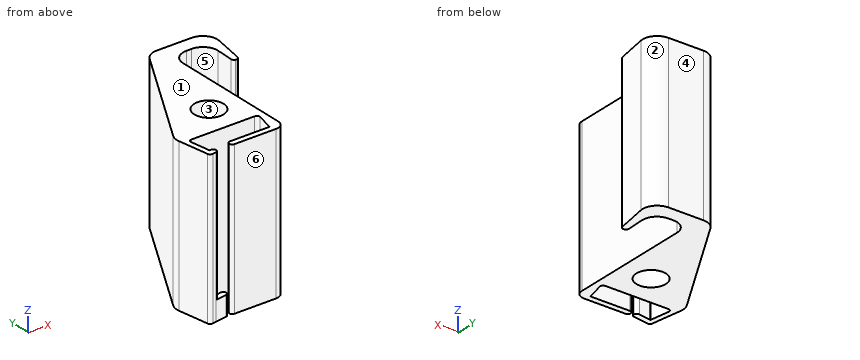
from build123d import *

# Parameters (mm, degrees)
F0_R     = 6.35
F1_DEPTH = 66.04
F3_DEPTH = 8.509


with BuildPart() as f1:
    # F0 (on Top) → F1 (new body)
    with BuildSketch(Plane.XY):
        with BuildLine():
            ThreePointArc((-22.546312, -25.022118), (-22.038436, -25.850898), (-21.093276, -26.077811))
            Line((-21.093276, -26.077811), (-19.546685, -25.832855))
            ThreePointArc((-19.546685, -25.832855), (-18.717905, -25.324978), (-18.490992, -24.379819))
            ThreePointArc((-18.490992, -24.379819), (-18.998869, -23.551039), (-19.944028, -23.324126))
            Line((-19.944028, -23.324126), (-20.432482, -23.40149))
            Line((-20.432482, -23.40149), (-21.789241, -14.835248))
            ThreePointArc((-21.789241, -14.835248), (-21.500592, -13.811777), (-20.534877, -13.366576))
            Line((-20.534877, -13.366576), (6.84281, -13.366576))
            ThreePointArc((6.84281, -13.366576), (7.841192, -13.851634), (8.076939, -14.936285))
            Line((8.076939, -14.936285), (6.237518, -22.510576))
            Line((6.237518, -22.510576), (-10.92632, -22.510576))
            ThreePointArc((-10.92632, -22.510576), (-11.824346, -22.882551), (-12.19632, -23.780576))
            ThreePointArc((-12.19632, -23.780576), (-11.824346, -24.678602), (-10.92632, -25.050576))
            Line((-10.92632, -25.050576), (7.188144, -25.050576))
            ThreePointArc((7.188144, -25.050576), (9.882221, -23.934653), (10.998144, -21.240576))
            Line((10.998144, -21.240576), (10.998144, 32.099424))
            ThreePointArc((10.998144, 32.099424), (12.858016, 36.589552), (17.348144, 38.449424))
            Line((17.348144, 38.449424), (19.672829, 38.449424))
            ThreePointArc((19.672829, 38.449424), (24.237179, 36.514082), (26.0193, 31.887757))
            Line((26.0193, 31.887757), (25.766103, 24.296054))
            ThreePointArc((25.766103, 24.296054), (26.040588, 23.464256), (26.788287, 23.007993))
            Line((26.788287, 23.007993), (26.945018, 22.976903))
            ThreePointArc((26.945018, 22.976903), (27.911116, 23.175751), (28.443527, 24.006066))
            Line((28.443527, 24.006066), (30.755673, 37.366601))
            ThreePointArc((30.755673, 37.366601), (29.356579, 42.538836), (24.498677, 44.799424))
            Line((24.498677, 44.799424), (9.376487, 44.799424))
            ThreePointArc((9.376487, 44.799424), (6.177033, 43.934494), (3.849171, 41.575328))
            Line((3.849171, 41.575328), (-23.920269, -7.527419))
            ThreePointArc((-23.920269, -7.527419), (-24.641712, -9.523939), (-24.664773, -11.646682))
            Line((-24.664773, -11.646682), (-22.546312, -25.022118))
        make_face()
        with Locations((-2.336856, 0.349424)):
            Circle(F0_R, mode=Mode.SUBTRACT)
    extrude(amount=F1_DEPTH)

    # F2 (on face) → F3 (join)
    with BuildSketch(Plane(origin=(0, 0, 0), x_dir=(1, 0, 0), z_dir=(0, 0, -1))):
        with BuildLine():
            ThreePointArc((-19.546685, 25.832855), (-18.490992, 24.379819), (-19.944028, 23.324126))
            Line((-19.944028, 23.324126), (-14.965174, 22.535553))
            ThreePointArc((-14.965174, 22.535553), (-14.020015, 22.762466), (-13.512138, 23.591246))
            ThreePointArc((-13.512138, 23.591246), (-13.739051, 24.536405), (-14.567831, 25.044282))
            Line((-14.567831, 25.044282), (-19.546685, 25.832855))
        make_face()
    extrude(amount=-F3_DEPTH)


solid = f1.part
Geometry: final body of the model. Coordinates: model frame, mm. Face numbers are marked on the shaded views. A direction names the side the tool comes from. Coordinates: 2 decimals unless noted, no trailing zeros. Loops run counter-clockwise (first coordinate to the right, second up) from the corner with the lowest first, then second, coordinate; pieces in that order, holes last. Notation, with made-up numbers: (68.5, 15) - (103.5, 15) arc R9 cw to (103.5, 31) - close; hole circle Ø11 at (-3, -4). An arc over 180 degrees is marked (long way). One line per question, with ' | ' between items. Start each with the question number.
(1) Ray query, L1, parallel to Y at x = -5, z = 4.5; L2, parallel to Y at x = 0.5, z = 55.5; L3, parallel to Y at x = -10, z = 61. Return the intervals inside material, ascending. Write a range as from..to.
(2) Cut plane B-B on y = 2. Output: boundary loops of the cut face in (x, z).
(3) Cut plane C-C on x = -10. Output: boundary loops of the cut face in (y, z).
(4) Reachability of the marked faces 4, 5 and 6 from +Z, -Z, +X, -X, +Y, -Y: full face, straight path, thin tool, end or side. Return the list, or none.
(5) Cut plane D-D on x = 18.5. Output: boundary loops of the cut face in (y, z).
(6) Draft query along X for the marked faces 1, 2 and 3. Return one class per face: +X half, -X half, draft (parallel to the pull), parting line (faces both ways), or undercut.
(7) First-contact query: pin 1 (3 mm diameter, centred on x = 20.5, z = 45, fed in from -Y); pin 2 (19 mm diameter, centred on x = -3.5, z = 41.5, fed in from +Y); pin 3 (2 mm diameter, centred on y = 2, z = 34.5, fed in from -X). Flat tips, straight axial feed; report the tip coordinate or a pass-through.
Here are the results:
1) L1: -25.05..-22.51, -13.37..-5.42, 6.11..25.93 | L2: -25.05..-22.51, -13.37..-5.33, 6.03..35.65 | L3: -25.05..-22.51, -13.37..17.09
2) outline: (-18.53, 0) - (-8.47, 0) - (-8.47, 66.04) - (-18.53, 66.04) - close; (3.79, 0) - (11, 0) - (11, 66.04) - (3.79, 66.04) - close
3) outline: (-25.05, 0) - (-22.51, 0) - (-22.51, 66.04) - (-25.05, 66.04) - close; (-13.37, 0) - (17.09, 0) - (17.09, 66.04) - (-13.37, 66.04) - close
4) face 4: +Z, -Z, +X, -X, +Y | face 5: +Z, -Z | face 6: +Z, -Z, +X, -Y
5) outline: (38.45, 0) - (44.8, 0) - (44.8, 66.04) - (38.45, 66.04) - close
6) face 1: draft | face 2: +X half | face 3: undercut
7) pin 1: y = 38.01 | pin 2: y = 43.83 | pin 3: x = -19.1
